```python
from build123d import *

# Parameters (mm, degrees)
SKETCH2_W           = 20
SKETCH2_H           = 28
BOSS_EXTRUDE1_DEPTH = 19
SKETCH3_W           = 12.5
SKETCH3_H           = 23.25
CUT_EXTRUDE1_DEPTH  = 16
SKETCH4_W           = 20
SKETCH4_H           = 19
BOSS_EXTRUDE3_DEPTH = 7
SKETCH5_W           = 9
SKETCH5_H           = 5
CUT_EXTRUDE2_DEPTH  = 31.033314835


with BuildPart() as part:
    # Sketch2 → Boss-Extrude1 (new body)
    with BuildSketch(Plane(origin=(0, 0, 0), x_dir=(1, 0, 0), z_dir=(0, 1, 0))):
        Rectangle(SKETCH2_W, SKETCH2_H)
    extrude(amount=BOSS_EXTRUDE1_DEPTH)

    # Sketch3 → Cut-Extrude1 (cut)
    with BuildSketch(Plane(origin=(0, 19, 0), x_dir=(1, 0, 0), z_dir=(0, 1, 0))):
        Rectangle(SKETCH3_W, SKETCH3_H)
    extrude(amount=-CUT_EXTRUDE1_DEPTH, mode=Mode.SUBTRACT)

    # Sketch4 → Boss-Extrude3 (add)
    with BuildSketch(Plane(origin=(0, 0, -14), x_dir=(-1, 0, 0), z_dir=(0, 0, -1))):
        with Locations((0, 9.5)):
            Rectangle(SKETCH4_W, SKETCH4_H)
    extrude(amount=BOSS_EXTRUDE3_DEPTH)

    # Sketch5 → Cut-Extrude2 (cut, through all)
    with BuildSketch(Plane.XZ):
        with Locations((0, -10.625)):
            Rectangle(SKETCH5_W, SKETCH5_H)
    extrude(amount=-CUT_EXTRUDE2_DEPTH, mode=Mode.SUBTRACT)


solid = part.part
```
Could you check a few things on this model? Use its own coordinates, in mm. A direction names the side the tool comes from. Round coordinates to 2 decimals unless told otherwise and drop trailing zeros. Order: outer loops, then holes, each group sorted by start corner. A loop starts at its lowest first (then second) coordinate and runs counter-clockwise, first axis right, second up. Notation, with made-up numbers: (78, 43) -> (137, 43) arc R18 ccw to (137, 63) -> close; hole circle Ø5 at (15.5, 44). An arc over 180 degrees is marked (long way). One line per question, with ' | ' between items.
Q1. If we section it at A-A on x = -0.75: Write out the boundary of the cut face in (y, z) (3 decimals).
Computed values:
outline: (0, -21) -> (19, -21) -> (19, -13.125) -> (0, -13.125) -> close; (0, -8.125) -> (3, -8.125) -> (3, 11.625) -> (19, 11.625) -> (19, 14) -> (0, 14) -> close
Q2. We'd pull the mould along X, two halves only. Please class faces 4 (the face through (-10, 9, -3)), 5 (the face through (-5, 11, -11.625)), 6 (the face through (7, 19, -3)): released by +X, released by -X, zero draft, split by the parting line, or undercut.
Computed values:
face 4: released by -X | face 5: undercut | face 6: zero draft
Q3. I'm going to push a flat-ended pin straight in: pin 1 (10 mm diameter, centred on x = 0, z = 3.5, fed in from +Y). Where does the tip first touch, or does it pass through?
Computed values:
pin 1: y = 3
Q4. If we section it at D-D on y = 2.25: Write out the boundary of the cut face in (x, z) (3 decimals), plus the area to 3 significant figures.
Computed values:
outline: (-10, -21) -> (10, -21) -> (10, 14) -> (-10, 14) -> close; hole (-4.5, -13.125) -> (4.5, -13.125) -> (4.5, -8.125) -> (-4.5, -8.125) -> close | area: 655 mm²
Q5. If I drill on line 1 (X direction, y = 3.25, z = 0); line 2 (Z direction, x = -5.75, y = 5.25) (3 decimals); line 3 (X direction, y = 1.5, z = -11.5), over which ranges is the centre line in solid material (lowest first)? Write a range as from..to.
Computed values:
line 1: -10..-6.25, 6.25..10 | line 2: -21..-11.625, 11.625..14 | line 3: -10..-4.5, 4.5..10
Q6. Which directions (+Z, -Z, +X, -X, +Y, -Y) give clear straight access to the entire face, cutting with the end or side of a thin tool? Please do faces 1 (the face through (4.5, 7, -12)), 2 (the face through (10, 9, -3)), 3 (the face through (0, 3, 0)).
Computed values:
face 1: +Y, -Y | face 2: +Z, -Z, +X, +Y, -Y | face 3: +Y
Q7. If we section it at C-C on z = 6.5: Write out the boundary of the cut face in (x, y).
Computed values:
outline: (-10, 0) -> (10, 0) -> (10, 19) -> (6.25, 19) -> (6.25, 3) -> (-6.25, 3) -> (-6.25, 19) -> (-10, 19) -> close
Q8. If we section it at B-B on y = 12.5: Write out the boundary of the cut face in (x, z) (3 decimals), plus the area to 3 significant figures.
Computed values:
outline: (-10, -21) -> (10, -21) -> (10, 14) -> (-10, 14) -> close; hole (-6.25, -11.625) -> (-4.5, -11.625) -> (-4.5, -13.125) -> (4.5, -13.125) -> (4.5, -11.625) -> (6.25, -11.625) -> (6.25, 11.625) -> (-6.25, 11.625) -> close | area: 396 mm²
